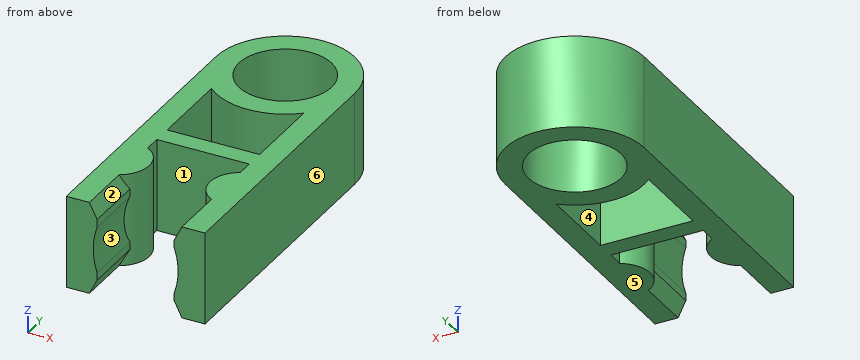
from build123d import *

# Parameters (mm, degrees)
EXTRUDE_1_DEPTH     = 6
SKETCH_2_R          = 3
CUT_EXTRUDE_1_DEPTH = 7
EXTRUDE_2_REACH     = 24.7


with BuildPart() as part:
    # 草图1 → 凸台-拉伸1 (new body)
    with BuildSketch(Plane.XY):
        with BuildLine():
            Line((-4.5, 0), (-4.5, -18.2))
            Line((-4.5, -18.2), (-3, -18.2))
            Line((-3, -18.2), (-3, -14.6))
            ThreePointArc((-3, -14.6), (-1.968245837, -12.85), (-3, -11.1))
            Line((-3, -11.1), (-3, -10))
            Line((-3, -10), (3, -10))
            Line((3, -10), (3, -11.1))
            ThreePointArc((3, -11.1), (1.968245837, -12.85), (3, -14.6))
            Line((3, -14.6), (3, -18.2))
            Line((3, -18.2), (4.5, -18.2))
            Line((4.5, -18.2), (4.5, 0))
            ThreePointArc((4.5, 0), (0, 4.5), (-4.5, 0))
        make_face()
    extrude(amount=EXTRUDE_1_DEPTH)

    # 草图2 → 切除-拉伸1 (cut, through all)
    with BuildSketch(Plane.XY):
        Circle(SKETCH_2_R)
        with BuildLine():
            Line((-3, -8.75), (-3, -3.354101966))
            ThreePointArc((-3, -3.354101966), (0, -4.5), (3, -3.354101966))
            Line((3, -3.354101966), (3, -8.75))
            Line((3, -8.75), (-3, -8.75))
        make_face()
    extrude(amount=CUT_EXTRUDE_1_DEPTH, mode=Mode.SUBTRACT)

    # 草图3 → 凸台-拉伸2 (add, up to next)
    with BuildSketch(Plane.XZ.offset(18.2), mode=Mode.PRIVATE) as extrude_2_sk1:
        with BuildLine():
            Line((-3, 6), (-3, 0))
            Line((-3, 0), (-2.5, 1))
            Line((-2.5, 1), (-2.5, 1.5))
            ThreePointArc((-2.5, 1.5), (-2.757359313, 3), (-2.5, 4.5))
            Line((-2.5, 4.5), (-2.5, 5))
            Line((-2.5, 5), (-3, 6))
        make_face()
    extrude_2_tool1 = extrude(extrude_2_sk1.sketch, amount=-EXTRUDE_2_REACH, mode=Mode.PRIVATE) - part.part
    add(extrude_2_tool1.solids().sort_by_distance((-2.809362, -18.2, 3))[0])
    # 草图3 → 凸台-拉伸2 (add, up to next)
    with BuildSketch(Plane.XZ.offset(18.2), mode=Mode.PRIVATE) as extrude_2_sk2:
        with BuildLine():
            Line((3, 0), (2.5, 1))
            Line((2.5, 1), (2.5, 1.5))
            ThreePointArc((2.5, 1.5), (2.757359313, 3), (2.5, 4.5))
            Line((2.5, 4.5), (2.5, 5))
            Line((2.5, 5), (3, 6))
            Line((3, 6), (3, 0))
        make_face()
    extrude_2_tool2 = extrude(extrude_2_sk2.sketch, amount=-EXTRUDE_2_REACH, mode=Mode.PRIVATE) - part.part
    add(extrude_2_tool2.solids().sort_by_distance((2.809362, -18.2, 3))[0])


solid = part.part
Source: CAD feature listing. Evaluate the final solid. Frame: model axes, mm. Face numbers are marked on the shaded views. A direction names the side the tool comes from. Coordinates: 2 decimals unless noted, no trailing zeros. Order: outer loops, then holes, each group sorted by start corner. A loop starts at its lowest first (then second) coordinate and runs counter-clockwise, first axis right, second up. Notation, with made-up numbers: M 13.25,-18.5 L 40.25,-18.5 A23 cw 40.25,-6.5 Z; hole C 46,37 d10. An arc over 180 degrees is marked long. Write each question's results on one line, items separated by ' | '. Start each with the question number.
1. Section A-A, the plane y = -6.5. Return the cut outline in (x, z).
2. Section C-C, the plane z = 2.25. Return the cut outline in (x, y).
3. Section B-B, the plane x = 0. Return the cut outline in (y, z).
4. Reachability of the marked faces 1, 2 and 3 from +Z, -Z, +X, -X, +Y, -Y: full face, straight path, thin tool, end or side. Return the list, or none.
5. Section D-D, the plane x = -1.25. Return the cut outline in (y, z), then the cut area to 3 significant figures.
6. Draft query along X for the marked faces 4, 5 and 6. Return one class per face: +X half, -X half, draft (parallel to the pull), parting line (faces both ways), or undercut.
7. Pin query (flat end, axial travel): pin 1 (1.5 mm diameter, centred on x = 3.5, z = 1, fed in from +Y); pin 2 (1 mm diameter, centred on x = 0, y = -6.5, fed in from -Z); pin 3 (1.8 mm diameter, centred on x = -1, z = 2, fed in from -Y). Return the tip coordinate at first contact, or that it passes through.
8. Material intervals for L1, parallel to Y at x = 0, z = 4.2; L2, parallel to X at y = 0, z = 2.1; L3, parallel to Y at x = -1.25, z = 1.5, sorted ascending.
Solution:
1) outline: M -4.5,0 L -3,0 L -3,6 L -4.5,6 Z; M 3,0 L 4.5,0 L 4.5,6 L 3,6 Z
2) outline: M -4.5,-18.2 L -2.69,-18.2 L -2.69,-14.39 A2 ccw -3,-11.1 L -3,-10 L 3,-10 L 3,-11.1 A2 ccw 2.69,-14.39 L 2.69,-18.2 L 4.5,-18.2 L 4.5,0 A4.5 ccw -4.5,0 Z; hole M -3,-8.75 L 3,-8.75 L 3,-3.35 A4.5 cw -3,-3.35 Z; hole C 0,0 d6
3) outline: M -10,0 L -8.75,0 L -8.75,6 L -10,6 Z; M -4.5,0 L -3,0 L -3,6 L -4.5,6 Z; M 3,0 L 4.5,0 L 4.5,6 L 3,6 Z
4) face 1: +Z, -Z | face 2: +Z, -Y | face 3: -Y
5) outline: M -10,0 L -8.75,0 L -8.75,6 L -10,6 Z; M -4.32,0 L -2.73,0 L -2.73,6 L -4.32,6 Z; M 2.73,0 L 4.32,0 L 4.32,6 L 2.73,6 Z | area: 26.6 mm²
6) face 4: undercut | face 5: draft | face 6: +X half
7) pin 1: y = 3.56 | pin 2: through | pin 3: y = -10
8) L1: -10 to -8.75, -4.5 to -3, 3 to 4.5 | L2: -4.5 to -3, 3 to 4.5 | L3: -10 to -8.75, -4.32 to -2.73, 2.73 to 4.32
